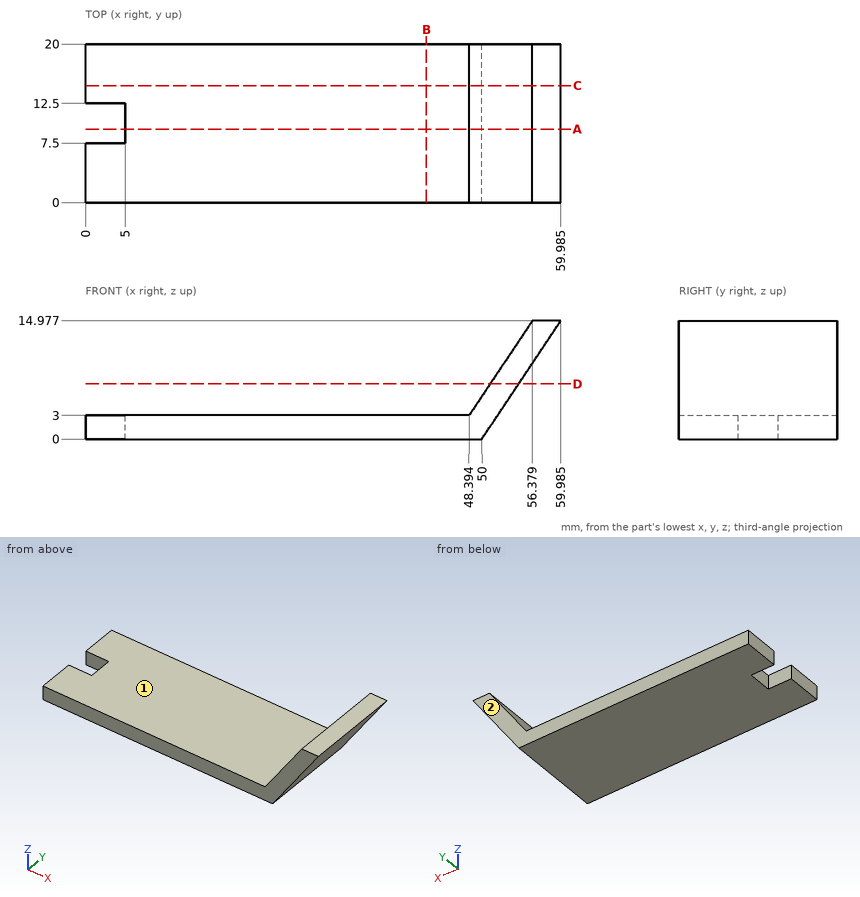
Study the drawing (mm; zero at the part's minimum x, y, z) and answer. A direction names the side the tool comes from. Round coordinates to 2 decimals unless told otherwise and drop trailing zeros. Write each loop counter-clockwise with the first axis right and the second up, starting at its lowest first coordinate (ties: lowest second). Pieces come first, ordered by that corner, then holes.
Q1. Find section C-C on y = 14.75. Determine the outline of the cut face in (x, z) (1 decimal).
Values:
outline: (0, 0) - (50, 0) - (60, 15) - (56.4, 15) - (48.4, 3) - (0, 3) - close
Q2. Find section A-A on y = 9.25. Determine the outline of the cut face in (x, z) (1 decimal).
Values:
outline: (5, 0) - (50, 0) - (60, 15) - (56.4, 15) - (48.4, 3) - (5, 3) - close
Q3. Flat-ended cylindrical pins translate along their axes: P1, Ø2, axis at y = 5, z = 10.5, coming from the -X side; P2, Ø6, axis at x = 25, y = 14, coming from the +Z side; P3, Ø5, axis at x = 14.5, z = 4.5, coming from the +Y side; P4, Ø3.5, axis at y = 9.5, z = 2, coming from the -X side. Find the tip coordinate at first contact, or state that the pin passes through.
Values:
P1: stops at x = 52.73
P2: stops at z = 3
P3: stops at y = 20
P4: stops at x = 5
Q4. Straight lines are drawn through the part: line 1 (Z direction, x = 28, y = 9.5); line 2 (X direction, y = 12.25, z = 7.75) (1 decimal); line 3 (X direction, y = 12.5, z = 3.5) (1 decimal). For each, find the intervals that lie inside material, in ascending order.
Values:
line 1: z = 0 to 3
line 2: x = 51.6 to 55.2
line 3: x = 48.7 to 52.3
Q5. A tool of negligible diameter and unlimited length cuts with its end or side. For the marked faces 1 and 2, from which of +Z, -Z, +X, -X, +Y, -Y can it reach the whole face along a straight path? Write none if from no direction.
Values:
face 1: +Z, -X, +Y, -Y
face 2: +Z, -Z, +X, -X, +Y
Q6. Find section B-B on x = 43. Determine the outline of the cut face in (y, z), and give its area (3 significant figures).
Values:
outline: (0, 0) - (20, 0) - (20, 3) - (0, 3) - close
area: 60.0 mm2
Q7. Find section D-D on z = 7. Determine the outline of the cut face in (x, y).
Values:
outline: (51.06, 0) - (54.67, 0) - (54.67, 20) - (51.06, 20) - close
